Could you check a few things on this model? Use its own coordinates, in mm. Give positions to 0.01 mm unless a question says otherwise; leave off trailing zeros. Order: outer loops, then holes, each group sorted by start corner. A loop starts at its lowest first (then second) coordinate and runs counter-clockwise, first axis right, second up.
from build123d import *

# Parameters (mm, degrees)
SKETCH_R      = 2.05
EXTRUDE_DEPTH = 5
CHAMFER_SIZE  = 2


with BuildPart() as part:
    # Sketch → Extrude (new body)
    with BuildSketch(Plane.XY):
        Polygon((0, 0), (0, 20), (20, 40), (40, 40), (60, 20), (60, 0), align=None)
        with Locations((10, 10)):
            Circle(SKETCH_R, mode=Mode.SUBTRACT)
        with Locations((50, 10)):
            Circle(SKETCH_R, mode=Mode.SUBTRACT)
        with Locations((30, 30)):
            Circle(SKETCH_R, mode=Mode.SUBTRACT)
    extrude(amount=EXTRUDE_DEPTH)

    # Chamfer
    chamfer_edges = [part.edges().sort_by_distance(p)[0] for p in [
        (0, 10, 5),
        (10, 30, 5),
        (30, 40, 5),
        (50, 30, 5),
        (60, 10, 5),
        (30, 0, 5),
    ]]
    chamfer(chamfer_edges, length=CHAMFER_SIZE)


solid = part.part
Item 1: We'd pull the mould along X, two halves only. Please class faces 1 (the flat face through (30, 40, 1)), 2 (the cylindrical face through (8.373, 8.753, 2.465)), 3 (the flat face through (59, 10, 4)): +X half, -X half, draft (parallel to the pull), parting line (faces both ways), or undercut.
Findings:
face 1: draft
face 2: undercut
face 3: +X half
Item 2: Please list where these lines run through material, in increasing order: line 1 along Y through (x, z) = (30, 2.65); line 2 along X through (y, z) = (11, 3.45); line 3 along Y through (x, z) = (10, 1.5).
Findings:
line 1: y = 0 to 27.95, 32.05 to 40
line 2: x = 0.45 to 8.21, 11.79 to 48.21, 51.79 to 59.55
line 3: y = 0 to 7.95, 12.05 to 30
Item 3: For pin 1 (3.5 mm diameter, centred on x = 10, y = 10, fed in from -Z); pin 2 (2 mm diameter, centred on y = 35.5, z = 4, fed in from +X), each with a flat end and sliding along its axis, tell me the tip position at first contact or that it passes through.
Findings:
pin 1: passes through
pin 2: stops at x = 44.82
Item 4: Imagine slicing it at B-B on y = 10. List the corners of the cut face in (x, z) for me.
Findings:
outline: (0, 0) - (7.95, 0) - (7.95, 5) - (2, 5) - (0, 3) - close; (12.05, 0) - (47.95, 0) - (47.95, 5) - (12.05, 5) - close; (52.05, 0) - (60, 0) - (60, 3) - (58, 5) - (52.05, 5) - close
Item 5: Imagine slicing it at C-C on z = 2.35. List the corners of the cut face in (x, y) for me, then the cut area to 3 significant figures.
Findings:
outline: (0, 0) - (60, 0) - (60, 20) - (40, 40) - (20, 40) - (0, 20) - close; hole circle Ø4.1 at (10, 10); hole circle Ø4.1 at (30, 30); hole circle Ø4.1 at (50, 10)
area: 1,960 mm2
Item 6: Imagine slicing it at D-D on y = 31. List the corners of the cut face in (x, z) for me, then the cut area to 3 significant figures.
Findings:
outline: (11, 0) - (28.21, 0) - (28.21, 5) - (13.83, 5) - (11, 3) - close; (31.79, 0) - (49, 0) - (49, 3) - (46.17, 5) - (31.79, 5) - close
area: 166 mm2
Item 7: Imagine slicing it at A-A on x = 30. List the corners of the cut face in (y, z) for me, then the cut area to 4 significant figures.
Findings:
outline: (0, 0) - (27.95, 0) - (27.95, 5) - (2, 5) - (0, 3) - close; (32.05, 0) - (40, 0) - (40, 3) - (38, 5) - (32.05, 5) - close
area: 175.5 mm2
